For this review, take the finished solid that the model builds, in its own axes (mm). A direction names the side the tool comes from. Coordinates: 2 decimals unless noted, no trailing zeros. Loops run counter-clockwise (first coordinate to the right, second up) from the corner with the lowest first, then second, coordinate; pieces in that order, holes last. Notation, with made-up numbers: M 88,9.5 L 115,9.5 A23 cw 115,41.5 Z; hole C 76.25,63.5 d7. An arc over 180 degrees is marked long. Answer as a JSON object with one key per item and string values. Group by question number.
Item 1: Wall thickness on L1, parallel to Y at x = 0, z = 133.2 (3 decimals); L2, parallel to X at y = 0.5, z = 100.5: over which ranges is each line inside the solid? List them lowest first. Write a range as from..to.
Item 2: Tool access review of faces 4 (the face through (7, 0, 135)), 5 (the face through (17, 10, 130)), 6 (the face through (-21.199, 6.676, 14.79)): name each direction out of +Z, -Z, +X, -X, +Y, -Y from which nothing blocks a thin tool from reaching the whole face with its end or side.
Item 3: Insertion check: pin 1 (6.5 mm diameter, centred on x = 17.32, y = -10, fed in from -Z); pin 2 (2 mm diameter, centred on x = -8.5, y = -0.5, fed in from -Z); pin 3 (4 mm diameter, centred on x = 0, y = 20, fed in from +Z); pin 4 (1.5 mm diameter, centred on y = -1.5, z = 51, fed in from +X). Each pin has a flat end and moves straight along its axis. Give the tip position at first contact, or say it passes through.
Item 4: Mouldability with a two-part tool opening along X and no side actions: class faces 1 (the face through (0, -5, 30)), 2 (the face through (-22, -7, 0)), 3 (the face through (-6.883, -30.995, 66.555)) as +X half, -X half, draft (parallel to the pull), parting line (faces both ways), or undercut.
Item 5: Add section A-A (y = 0). State the section outline as (x, z) points (3 decimals).
Item 6: Add section D-D (x = 10). State the section outline as (y, z) points, then the cut area to 3 significant figures.
Item 7: Add section C-C (z = 63.5). State the section outline as (x, y) points (3 decimals).
Item 8: Add section B-B (x = 0). State the section outline as (y, z) points (3 decimals), then the cut area to 3 significant figures.
from build123d import *

# Parameters (mm, degrees)
SKETCH2_R           = 31.75
BOSS_EXTRUDE1_DEPTH = 135
SKETCH3_R           = 3.815
CUT_EXTRUDE1_DEPTH  = 135
SKETCH5_R           = 22.225
CUT_EXTRUDE2_DEPTH  = 30
SKETCH6_R           = 2.5
CUT_EXTRUDE3_DEPTH  = 5
SKETCH6_3_R         = 2.5
CUT_EXTRUDE4_DEPTH  = 5


with BuildPart() as part:
    # Sketch2 → Boss-Extrude1 (new body)
    with BuildSketch(Plane.XY):
        Circle(SKETCH2_R)
    extrude(amount=BOSS_EXTRUDE1_DEPTH)

    # Sketch3 → Cut-Extrude1 (cut)
    with BuildSketch(Plane(origin=(0, 0, 0), x_dir=(-1, 0, 0), z_dir=(0, 0, -1))):
        Circle(SKETCH3_R)
    extrude(amount=-CUT_EXTRUDE1_DEPTH, mode=Mode.SUBTRACT)

    # Sketch5 → Cut-Extrude2 (cut)
    with BuildSketch(Plane(origin=(0, 0, 0), x_dir=(-1, 0, 0), z_dir=(0, 0, -1))):
        Circle(SKETCH5_R)
    extrude(amount=-CUT_EXTRUDE2_DEPTH, mode=Mode.SUBTRACT)

    # Sketch6 → Cut-Extrude3 (cut)
    with BuildSketch(Plane.XY.offset(135)):
        with Locations((0, 20)):
            Circle(SKETCH6_R)
    extrude(amount=-CUT_EXTRUDE3_DEPTH, mode=Mode.SUBTRACT)

    # Sketch6<3> → Cut-Extrude4 (cut)
    with BuildSketch(Plane.XY.offset(135)):
        with Locations((0, 20)):
            Circle(SKETCH6_3_R)
        with Locations((17.320508076, 10)):
            Circle(SKETCH6_3_R)
        with Locations((17.320508076, -10)):
            Circle(SKETCH6_3_R)
        with Locations((0, -20)):
            Circle(SKETCH6_3_R)
        with Locations((-17.320508076, -10)):
            Circle(SKETCH6_3_R)
        with Locations((-17.320508076, 10)):
            Circle(SKETCH6_3_R)
    extrude(amount=-CUT_EXTRUDE4_DEPTH, mode=Mode.SUBTRACT)


solid = part.part
From the geometry:
{
 "1": {"L1": "y = -31.75..-22.5, -17.5..-3.815, 3.815..17.5, 22.5..31.75", "L2": "x = -31.75..-3.78, 3.78..31.75"},
 "2": {"face 4": "+Z, +X, -X, +Y, -Y", "face 5": "+Z", "face 6": "-Z"},
 "3": {"pin 1": "stops at z = 0", "pin 2": "stops at z = 30", "pin 3": "stops at z = 130", "pin 4": "stops at x = 31.74"},
 "4": {"face 1": "undercut", "face 2": "draft", "face 3": "parting line"},
 "5": {"outline": "M -31.75,0 L -22.225,0 L -22.225,30 L -3.815,30 L -3.815,135 L -31.75,135 Z; M 3.815,30 L 22.225,30 L 22.225,0 L 31.75,0 L 31.75,135 L 3.815,135 Z"},
 "6": {"outline": "M -30.13,0 L -19.85,0 L -19.85,30 L 19.85,30 L 19.85,0 L 30.13,0 L 30.13,135 L -30.13,135 Z", "area": "6,950 mm²"},
 "7": {"outline": "C 0,0 d63.5; hole C 0,0 d7.63"},
 "8": {"outline": "M -31.75,0 L -22.225,0 L -22.225,30 L -3.815,30 L -3.815,135 L -17.5,135 L -17.5,130 L -22.5,130 L -22.5,135 L -31.75,135 Z; M 3.815,30 L 22.225,30 L 22.225,0 L 31.75,0 L 31.75,135 L 22.5,135 L 22.5,130 L 17.5,130 L 17.5,135 L 3.815,135 Z", "area": "6,390 mm²"}
}
